from build123d import *

# Parameters (mm, degrees)
BOSS_EXTRUDE1_DEPTH = 23
SKETCH2_R           = 3.5
BOSS_EXTRUDE2_DEPTH = 6
FILLET3_R           = 2
FILLET4_R           = 2
FILLET5_R           = 2
FILLET6_R           = 2
FILLET7_R           = 2
FILLET8_R           = 2
CUT_EXTRUDE2_START  = -6
CUT_EXTRUDE2_DEPTH  = 6


with BuildPart() as part:
    # Sketch1 → Boss-Extrude1 (new body)
    with BuildSketch(Plane(origin=(0, 0, 0), x_dir=(0, 0, -1), z_dir=(1, 0, 0))):
        Polygon((0, 0), (0, 16), (22, 16), (22, 47), (42, 47), (42, 0), align=None)
    extrude(amount=BOSS_EXTRUDE1_DEPTH)

    # Sketch2 → Boss-Extrude2 (add)
    with BuildSketch(Plane(origin=(0, 0, 0), x_dir=(-1, 0, 0), z_dir=(0, -1, 0))):
        with Locations(Location((-11.5, 10.5, 0), (0, 0, 270))):
            Circle(SKETCH2_R)
    extrude(amount=BOSS_EXTRUDE2_DEPTH)

    # Fillet3
    fillet3_edges = [part.edges().sort_by_distance(p)[0] for p in [
        (23, 8, 0),
    ]]
    fillet(fillet3_edges, radius=FILLET3_R)

    # Fillet4
    fillet4_edges = [part.edges().sort_by_distance(p)[0] for p in [
        (0, 8, 0),
    ]]
    fillet(fillet4_edges, radius=FILLET4_R)

    # Fillet5
    fillet5_edges = [part.edges().sort_by_distance(p)[0] for p in [
        (23, 23.5, -42),
    ]]
    fillet(fillet5_edges, radius=FILLET5_R)

    # Fillet6
    fillet6_edges = [part.edges().sort_by_distance(p)[0] for p in [
        (0, 23.5, -42),
    ]]
    fillet(fillet6_edges, radius=FILLET6_R)

    # Fillet7
    fillet7_edges = [part.edges().sort_by_distance(p)[0] for p in [
        (0, 31.5, -22),
    ]]
    fillet(fillet7_edges, radius=FILLET7_R)

    # Fillet8
    fillet8_edges = [part.edges().sort_by_distance(p)[0] for p in [
        (23, 31.5, -22),
    ]]
    fillet(fillet8_edges, radius=FILLET8_R)

    # Sketch3 → Cut-Extrude2 (cut)
    with BuildSketch(Plane.XZ.offset(6).offset(CUT_EXTRUDE2_START)):
        with BuildLine():
            Line((9.050510257, -13), (13.949489743, -13))
            ThreePointArc((13.949489743, -13), (11.5, -14), (9.050510257, -13))
        make_face()
        with BuildLine():
            Line((9.050510257, -8), (13.949489743, -8))
            ThreePointArc((13.949489743, -8), (11.5, -7), (9.050510257, -8))
        make_face()
    extrude(amount=CUT_EXTRUDE2_DEPTH, mode=Mode.SUBTRACT)


solid = part.part
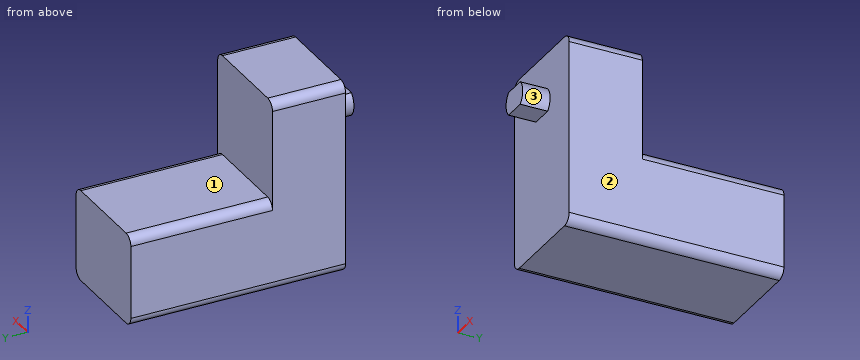
Model file for the job. Use its own axes, mm. Face numbers are marked on the shaded views. A direction names the side the tool comes from. Round coordinates to 2 decimals unless told otherwise and drop trailing zeros. Order: outer loops, then holes, each group sorted by start corner. A loop starts at its lowest first (then second) coordinate and runs counter-clockwise, first axis right, second up.
(1) Drill centre lines: line 1 (Y direction, x = 11.5, z = -16); line 2 (Z direction, x = 12.75, y = -4); line 3 (Z direction, x = 17.75, y = 34.5). Where is each one in solid material? Low to high.
(2) 3-axis set-ups, long thin cutter, end or side, ignore diameter. For the marked faces 1, 2 and 3: which of +Z, -Z, +X, -X, +Y, -Y reach the whole face in a straight line?
(3) Band-saw the part on A-A (y = 24). List the corners of the cut face in (x, z).
(4) Band-saw the part on B-B (x = 20). List the corners of the cut face in (y, z).
(5) Pin check, flat tips, straight feed: pin 1 (6 mm diameter, centred on x = 3.5, z = -14.5, fed in from -Y); pin 2 (1.5 mm diameter, centred on x = 12, y = -3, fed in from +Z); pin 3 (7 mm diameter, centred on x = 10, z = -9, fed in from +Y); pin 4 (8 mm diameter, centred on x = 15, z = -18.5, fed in from +Y). Stop position of each tip, or through.
(6) Band-saw the part on C-C (z = -36). List the corners of the cut face in (x, y), then the cut area to 3 significant figures.
(7) Band-saw the part on D-D (x = 10.5). List the corners of the cut face in (y, z).
Verdict:
1. line 1: y = 0 to 16
1. line 2: z = -13 to -8
1. line 3: z = -42 to -22
2. face 1: +Z, +X, -X, +Y
2. face 2: +Z, -Z, +X, +Y, -Y
2. face 3: +X, -Y
3. outline: (0, -40) arc R2 ccw to (2, -42) - (21, -42) arc R2 ccw to (23, -40) - (23, -24) arc R2 ccw to (21, -22) - (2, -22) arc R2 ccw to (0, -24) - close
4. outline: (0, -42) - (47, -42) - (47, -22) - (16, -22) - (16, 0) - (0, 0) - close
5. pin 1: stops at y = 0
5. pin 2: stops at z = -8
5. pin 3: stops at y = 16
5. pin 4: stops at y = 47
6. outline: (0, 0) - (23, 0) - (23, 47) - (0, 47) - close
6. area: 1,080 mm2
7. outline: (-6, -13) - (0, -13) - (0, -42) - (47, -42) - (47, -22) - (16, -22) - (16, 0) - (0, 0) - (0, -8) - (-6, -8) - close
